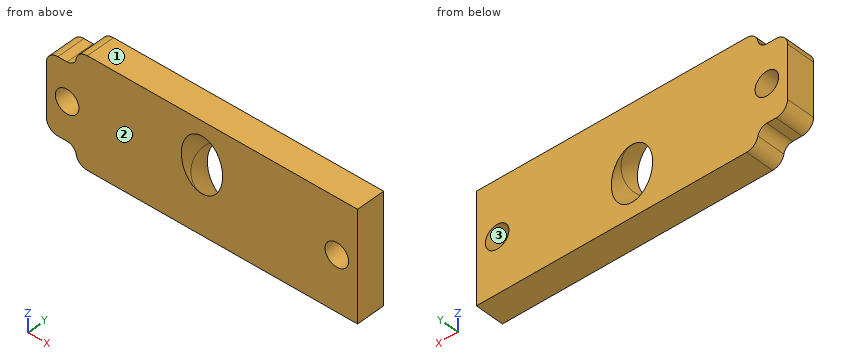
```python
from build123d import *

# Parameters (mm, degrees)
SKETCH2_W                      = 68.58
SKETCH2_H                      = 24.13
SKETCH2_R                      = 2.6
BOSS_EXTRUDE1_DEPTH            = 6.35
CUT_EXTRUDE1_DEPTH             = 7.35
FILLET3_R                      = 2.54
CUT_EXTRUDE2_REACH             = 12.372
SKETCH7_R                      = 4.55
CUT_EXTRUDE2_DIRECTION_2_REACH = 12.372


with BuildPart() as part:
    # Sketch2 → Boss-Extrude1 (new body)
    with BuildSketch(Plane(origin=(0, 0, 0), x_dir=(1, 0, 0), z_dir=(0, 1, 0))):
        with Locations((34.29, 12.065)):
            Rectangle(SKETCH2_W, SKETCH2_H)
        with Locations((4.57, 12.065)):
            Circle(SKETCH2_R, mode=Mode.SUBTRACT)
        with Locations((64.01, 12.065)):
            Circle(SKETCH2_R, mode=Mode.SUBTRACT)
    extrude(amount=BOSS_EXTRUDE1_DEPTH)

    # Sketch3 → Cut-Extrude1 (cut, through all)
    with BuildSketch(Plane(origin=(0, 6.35, 0), x_dir=(1, 0, 0), z_dir=(0, 1, 0))):
        with BuildLine():
            Line((4.57, 3.715), (0, 3.715))
            Line((0, 3.715), (0, 0))
            Line((0, 0), (6.57, 0))
            Line((6.57, 0), (6.57, 1.715))
            ThreePointArc((6.57, 1.715), (5.984213562, 3.129213562), (4.57, 3.715))
        make_face()
        with BuildLine():
            ThreePointArc((4.57, 20.415), (5.984213562, 21.000786438), (6.57, 22.415))
            Line((6.57, 22.415), (6.57, 24.13))
            Line((6.57, 24.13), (0, 24.13))
            Line((0, 24.13), (0, 20.415))
            Line((0, 20.415), (4.57, 20.415))
        make_face()
    extrude(amount=-CUT_EXTRUDE1_DEPTH, mode=Mode.SUBTRACT)

    # Fillet3
    fillet3_edges = [part.edges().sort_by_distance(p)[0] for p in [
        (6.57, 3.175, 0),
        (0, 3.175, -3.715),
        (0, 3.175, -20.415),
        (6.57, 3.175, -24.13),
    ]]
    fillet(fillet3_edges, radius=FILLET3_R)

    # Sketch7 → Cut-Extrude2 (cut, up to next)
    with BuildSketch(Plane(origin=(0, 7.768502242, -6.872990202), x_dir=(-1, 0, 0), z_dir=(0, -0.748955721, 0.662620048)), mode=Mode.PRIVATE) as cut_extrude2_sk1:
        with Locations((-34.29, 6.932332118)):
            Circle(SKETCH7_R)
    cut_extrude2_tool1 = extrude(cut_extrude2_sk1.sketch, amount=-CUT_EXTRUDE2_REACH, mode=Mode.PRIVATE) & part.part
    add(cut_extrude2_tool1.solids().sort_by_distance((34.29, 3.175, -12.065))[0], mode=Mode.SUBTRACT)

    # Sketch7 → Cut-Extrude2 direction 2 (cut, up to next)
    with BuildSketch(Plane(origin=(0, 7.768502242, -6.872990202), x_dir=(-1, 0, 0), z_dir=(0, -0.748955721, 0.662620048)), mode=Mode.PRIVATE) as cut_extrude2_direction_2_sk1:
        with Locations((-34.29, 6.932332118)):
            Circle(SKETCH7_R)
    cut_extrude2_direction_2_tool1 = extrude(cut_extrude2_direction_2_sk1.sketch, amount=CUT_EXTRUDE2_DIRECTION_2_REACH, mode=Mode.PRIVATE) & part.part
    add(cut_extrude2_direction_2_tool1.solids().sort_by_distance((34.29, 3.175, -12.065))[0], mode=Mode.SUBTRACT)


solid = part.part
```
Read the model definition and answer for the solid it produces. Units are mm, in the model's axes. Face numbers are marked on the shaded views. Give positions to 0.01 mm unless a question says otherwise; leave off trailing zeros. Write each loop counter-clockwise with the first axis right and the second up, starting at its lowest first coordinate (ties: lowest second). Pieces come first, ordered by that corner, then holes. Notation, with made-up numbers: (-10, -30) -> (-5, -30) arc R7 cw to (-5, -18) -> close; hole circle Ø3 at (27, -25.75). An arc over 180 degrees is marked (long way). Answer as a JSON object with one key per item and string values.
1) For a pull along Z with two mould halves and no side action, classify the marked faces 1, 2 and 3 as pulls with the +Z half, pulls with the -Z half, needs draft (parallel to the pull), parting line crosses it, or undercut.
Findings below:
{"face 1": "pulls with the +Z half", "face 2": "needs draft", "face 3": "undercut"}
2) Section A-A on x = 64.01 is taken. Write down the section's boundary in (y, z) (3 decimals), then the cut area to 3 significant figures.
Findings below:
{"outline": "(0, -24.13) -> (6.35, -24.13) -> (6.35, -14.665) -> (0, -14.665) -> close; (0, -9.465) -> (6.35, -9.465) -> (6.35, 0) -> (0, 0) -> close", "area": "120 mm^2"}
3) Flat-ended cylindrical pins translate along their axes: pin 1 Ø0.6 at (x, y) = (3.5, 3.5) entering from +Z (3 decimals); pin 2 Ø1 at (x, y) = (4, 4.5) entering from -Z (3 decimals); pin 3 Ø4 at (x, z) = (64.01, -12.065) entering from -Y; pin 4 Ø3 at (x, z) = (34.5, -19) entering from +Y. Find the tip coordinate at first contact, or state that the pin passes through.
Findings below:
{"pin 1": "stops at z = -3.715", "pin 2": "stops at z = -20.415", "pin 3": "passes through", "pin 4": "stops at y = 5.86"}
4) Section C-C on z = -14 is taken. Count the separate pieces of the cut face and the enclosed holes in it, then the cut area to 3 significant figures.
Findings below:
{"separate pieces": "4", "enclosed holes": "0", "area": "339 mm^2"}
5) Straight lines are drawn through the part: probe 1 along Z at (x, y) = (4.5, 3.5) (3 decimals); probe 2 along Z at (x, y) = (64.01, 2) (3 decimals); probe 3 along X at (y, z) = (4.25, -15.5). For each, find the intervals that lie inside material, in ascending order. Write a range as from..to.
Findings below:
{"probe 1": "z = -20.415..-14.664, -9.466..-3.715", "probe 2": "z = -24.13..-14.665, -9.465..0", "probe 3": "x = 0..30.14, 38.44..68.58"}
6) Section B-B on x = 32.5 is taken. Write down the section's boundary in (y, z), then the cut area to 3 significant figures.
Findings below:
{"outline": "(0, -24.13) -> (6.35, -24.13) -> (6.35, -20.46) -> (0, -14.84) -> close; (0, -3.67) -> (6.35, -9.29) -> (6.35, 0) -> (0, 0) -> close", "area": "82.3 mm^2"}
